Geometry: final body of the model. Coordinates: model frame, mm. A direction names the side the tool comes from. Round coordinates to 2 decimals unless told otherwise and drop trailing zeros. Order: outer loops, then holes, each group sorted by start corner. A loop starts at its lowest first (then second) coordinate and runs counter-clockwise, first axis right, second up. Notation, with made-up numbers: M -20.75,-30.5 L 29.25,-30.5 A21 cw 29.25,-0.5 Z; hole C 13.25,9.25 d3. An arc over 180 degrees is marked long. Return JSON: item names as keys, results as strings. Group by question number.
Q1. Access query for faces 4 (the face through (-89.873, 325.229, 12.325)), 5 (the face through (1857.419, 549.645, 12.325)). Directions: +Z, -Z, +X, -X, +Y, -Y. A direction counts if a zero-diameter tool reaches every point of the face in a straight line with its end or side. Return the directions, or none.
Q2. Ray query, probe 1 along X at (y, z) = (188, 23.25); probe 2 along X at (y, z) = (329, 3); probe 3 along X at (y, z) = (363.5, 18.5). Return the intervals inside material, ascending.
Q3. Contact query for flat-ended pins moving along their axis: pin 1 (7.5 mm diameter, centred on y = 423, z = 11, fed in from -X); pin 2 (4 mm diameter, centred on y = 364.5, z = 16, fed in from +X); pin 3 (12.5 mm diameter, centred on y = 319.5, z = 14.5, fed in from +X). Output: stop coordinate, or through.
Q4. Cut plane B-B on x = -300. Output: boundary loops of the cut face in (y, z).
Q5. Mould query, pull axis Y, two halves, no side actions, for faces 1 (the face through (-349.645, 557.419, 12.325)), 2 (the face through (733, 355, 0)), 3 (the face through (1608, 308, 12)). Classes: released by +Y, released by -Y, zero draft, split by the parting line, or undercut.
Q6. Cut plane D-D on x = 1652. Output: boundary loops of the cut face in (y, z).
Q7. Cut plane C-C on z = 21.25. Output: boundary loops of the cut face in (x, y).
Q8. Cut plane A-A on y = 150. Output: boundary loops of the cut face in (x, z).
```python
from build123d import *

# Parameters (mm, degrees)
F0_R     = 75
F0_W     = 25
F0_H     = 300
F1_DEPTH = 25


with BuildPart() as f1:
    # F0 (on Top) → F1 (new body)
    with BuildSketch(Plane.XY):
        with BuildLine():
            Line((-500, 200), (-500, 0))
            Line((-500, 0), (2000, 0))
            Line((2000, 0), (2000, 200))
            ThreePointArc((2000, 200), (1853.553391, 553.553391), (1500, 700))
            Line((1500, 700), (0, 700))
            ThreePointArc((0, 700), (-353.553391, 553.553391), (-500, 200))
        make_face()
        with Locations((-300, 150)):
            Circle(F0_R, mode=Mode.SUBTRACT)
        Polygon((17.67767, 217.67767), (0, 200), (-212.132034, 412.132034), (-194.454365, 429.809704), align=None, mode=Mode.SUBTRACT)
        with Locations((1800, 150)):
            Circle(F0_R, mode=Mode.SUBTRACT)
        with Locations((750, 350)):
            Rectangle(F0_W, F0_H, mode=Mode.SUBTRACT)
        Polygon((1712.132034, 412.132034), (1500, 200), (1482.32233, 217.67767), (1694.454365, 429.809704), align=None, mode=Mode.SUBTRACT)
    extrude(amount=F1_DEPTH)


solid = f1.part
```
Result sheet:
{
 "1": {"face 4": "+Z, -Z", "face 5": "+Z, -Z, +X, +Y"},
 "2": {"probe 1": "x = -500 to -364.66, -235.34 to 1735.34, 1864.66 to 2000", "probe 2": "x = -483.07 to -129, -93.64 to 737.5, 762.5 to 1593.64, 1629 to 1983.07", "probe 3": "x = -472.51 to -163.5, -128.14 to 737.5, 762.5 to 1628.14, 1663.5 to 1972.51"},
 "3": {"pin 1": "stops at x = -449.37", "pin 2": "stops at x = 1972.86", "pin 3": "stops at x = 1987.01"},
 "4": {"outline": "M 0,0 L 75,0 L 75,25 L 0,25 Z; M 225,0 L 600,0 L 600,25 L 225,25 Z"},
 "5": {"face 1": "released by +Y", "face 2": "zero draft", "face 3": "undercut"},
 "6": {"outline": "M 0,0 L 352,0 L 352,25 L 0,25 Z; M 387.36,0 L 676.34,0 L 676.34,25 L 387.36,25 Z"},
 "7": {"outline": "M -500,0 L 2000,0 L 2000,200 A500 ccw 1500,700 L 0,700 A500 ccw -500,200 Z; hole C -300,150 d150; hole M -212.13,412.13 L 0,200 L 17.68,217.68 L -194.45,429.81 Z; hole M 737.5,200 L 762.5,200 L 762.5,500 L 737.5,500 Z; hole M 1482.32,217.68 L 1500,200 L 1712.13,412.13 L 1694.45,429.81 Z; hole C 1800,150 d150"},
 "8": {"outline": "M -500,0 L -375,0 L -375,25 L -500,25 Z; M -225,0 L 1725,0 L 1725,25 L -225,25 Z; M 1875,0 L 2000,0 L 2000,25 L 1875,25 Z"}
}
